For this review, take the finished solid that the model builds, in its own axes (mm). A direction names the side the tool comes from. Coordinates: 2 decimals unless noted, no trailing zeros. Loops run counter-clockwise (first coordinate to the right, second up) from the corner with the lowest first, then second, coordinate; pieces in that order, holes last. Notation, with made-up numbers: M 19,80.25 L 39,80.25 A13 cw 39,102.25 Z; hole C 83,-31 d10. An arc over 180 degrees is marked long. Answer as a JSON object with one key per item and string values. Group by question number.
Item 1: Insertion check: pin 1 (10.5 mm diameter, centred on y = 12.5, z = 0, fed in from -X); pin 2 (5.5 mm diameter, centred on y = 12.5, z = 0, fed in from +X); pin 3 (1 mm diameter, centred on x = 22.5, y = -82.5, fed in from +Z). Each pin has a flat end and moves straight along its axis. Give the tip position at first contact, or say it passes through.
Item 2: Mouldability with a two-part tool opening along Z and no side actions: class faces 1 (the face through (0.422, 12.113, -73.344)), 2 (the face through (14.524, -67.751, 65.407)), 3 (the face through (9.373, -76.644, -71.387)) as +Z half, -Z half, draft (parallel to the pull), parting line (faces both ways), or undercut.
Item 3: Wall thickness on L1, parallel to X at y = -82, z = 0; L2, parallel to X at y = 7, z = 0; L3, parallel to Y at x = 78, z = 0: over which ranges is each line inside the solid? List them lowest first. Write a range as from..to.
Item 4: Add section A-A (y = -87.5). State the section outline as (x, z) points, then the cut area to 3 significant figures.
Item 5: Tool access review of faces 4 (the face through (-81.08, 15.72, -0.72)), 5 (the face through (0.72, 15.72, -81.08)), 6 (the face through (15.39, 12.68, 69.31)): name each direction out of +Z, -Z, +X, -X, +Y, -Y from which nothing blocks a thin tool from reaching the whole face with its end or side.
from build123d import *

# Parameters (mm, degrees)
CIRPATTERN1_COUNT = 4


with BuildPart() as part:
    # Sketch1 → Revolve1 (revolve)
    with BuildSketch(Plane.XY):
        Polygon((-71, 0), (-71, 25), (-87, 25), (-87, 0), (-92, 0), (-92, -30), (-72, -30), (-72, -122), (-67, -122), (-67, -15), align=None)
    revolve(axis=Axis((0, 25, 0), (0, -1, 0)))

    # Sketch6 → M6 Clearance Hole2 (revolve, cut)
    with BuildSketch(Plane(origin=(-87, 12.5, 0), x_dir=(0, 0, 1), z_dir=(0, 1, 0))):
        Polygon((0, 0), (0, 14), (3.3, 12.017159957), (3.3, 0), align=None)
    m6_clearance_hole2 = revolve(axis=Axis((-93.35, 12.5, 0), (1, 0, 0)), mode=Mode.SUBTRACT)

    # CirPattern1: M6 Clearance Hole2 ×4 about axis
    cirpattern1_axis = Axis((0, 25, 0), (0, 1, 0))
    for i in range(1, CIRPATTERN1_COUNT):
        add(m6_clearance_hole2.rotate(cirpattern1_axis, i * 360 / CIRPATTERN1_COUNT), mode=Mode.SUBTRACT)


solid = part.part
From the geometry:
{
 "1": {"pin 1": "stops at x = -87", "pin 2": "stops at x = 74.65", "pin 3": "stops at z = 68.56"},
 "2": {"face 1": "-Z half", "face 2": "undercut", "face 3": "parting line"},
 "3": {"L1": "x = -72..-67, 67..72", "L2": "x = -87..-71, 71..87", "L3": "y = -30..9.2, 15.8..25"},
 "4": {"outline": "C 0,0 d144; hole C 0,0 d134", "area": "2,180 mm²"},
 "5": {"face 4": "-X", "face 5": "-Z", "face 6": "+Y"}
}
